from build123d import *

# Parameters (mm, degrees)
ESBO_O1_W             = 42
ESBO_O1_H             = 42
FLANGE_BASE1_DEPTH    = 9.55
CORTE_EXTRUS_O2_DEPTH = 32.196193678
ESBO_O4_R             = 4.8
CORTE_EXTRUS_O4_DEPTH = 32.196193678
ESBO_O16_R            = 2
CORTE_EXTRUS_O6_DEPTH = 3
ESBO_O19_R            = 1.6
CORTE_EXTRUS_O7_DEPTH = 31.412209719


# Sheet-metal steps are written as plain solids
with BuildPart() as part:
    # Esboço1 → Flange-base1 (new body)
    with BuildSketch(Plane(origin=(0, 0, 0), x_dir=(1, 0, 0), z_dir=(0, 1, 0))):
        Rectangle(ESBO_O1_W, ESBO_O1_H)
    extrude(amount=-FLANGE_BASE1_DEPTH)

    # Esboço3 → Corte-extrusão2 (cut, through all)
    with BuildSketch(Plane.XZ.offset(9.55)):
        Polygon((-21, 16.757359313), (-16.757359313, 21), (-21, 21), align=None)
        Polygon((-21, -21), (-21, -16.757359313), (-16.757359313, -21), align=None)
        Polygon((21, -21), (21, -16.757359313), (16.757359313, -21), align=None)
        Polygon((21, 16.757359313), (21, 21), (16.757359313, 21), align=None)
    extrude(amount=-CORTE_EXTRUS_O2_DEPTH, mode=Mode.SUBTRACT)

    # Esboço4 → Corte-extrusão4 (cut, through all)
    with BuildSketch(Plane.XZ.offset(9.55)):
        with Locations(Location((0, 0, 0), (0, 0, 270))):
            Circle(ESBO_O4_R)
    extrude(amount=-CORTE_EXTRUS_O4_DEPTH, mode=Mode.SUBTRACT)

    # Esboço16 → Corte-extrusão6 (cut)
    with BuildSketch(Plane.XZ.offset(9.55)):
        with Locations(Location((-15.5, -15.5, 0), (0, 0, 270))):
            Circle(ESBO_O16_R)
        with Locations(Location((-15.5, 15.5, 0), (0, 0, 270))):
            Circle(ESBO_O16_R)
        with Locations(Location((15.5, 15.5, 0), (0, 0, 270))):
            Circle(ESBO_O16_R)
        with Locations(Location((15.5, -15.5, 0), (0, 0, 270))):
            Circle(ESBO_O16_R)
    extrude(amount=-CORTE_EXTRUS_O6_DEPTH, mode=Mode.SUBTRACT)

    # Esboço19 → Corte-extrusão7 (cut, through all)
    with BuildSketch(Plane.XZ.offset(6.55)):
        with Locations(Location((15.5, -15.5, 0), (0, 0, 270))):
            Circle(ESBO_O19_R)
        with Locations(Location((-15.5, -15.5, 0), (0, 0, 270))):
            Circle(ESBO_O19_R)
        with Locations(Location((15.5, 15.5, 0), (0, 0, 270))):
            Circle(ESBO_O19_R)
        with Locations(Location((-15.5, 15.5, 0), (0, 0, 270))):
            Circle(ESBO_O19_R)
    extrude(amount=-CORTE_EXTRUS_O7_DEPTH, mode=Mode.SUBTRACT)


solid = part.part
Geometry check sheet. Reference: the model listing, model coordinates, mm. A direction names the side the tool comes from. Round coordinates to 2 decimals unless told otherwise and drop trailing zeros. Write each loop counter-clockwise with the first axis right and the second up, starting at its lowest first coordinate (ties: lowest second). Pieces come first, ordered by that corner, then holes. Notation, with made-up numbers: (6, 34.25) -> (35, 34.25) arc R8 ccw to (35, 42.25) -> close; hole circle Ø8 at (36.25, 83). An arc over 180 degrees is marked (long way). One line per item, written item: value. Start each with the question number.
(1) Go/stop test with flat-tipped pins: pin 1 Ø11 at (x, z) = (0, 0) entering from -Y; pin 2 Ø3.5 at (x, z) = (15.5, 15.5) entering from -Y; pin 3 Ø1.2 at (x, z) = (16, 16) entering from -Y (3 decimals); pin 4 Ø1.2 at (x, z) = (-15, 16.5) entering from -Y. Record where each tip stops, or that it passes through.
(2) Access from +Z, -Z, +X, -X, +Y, -Y to the whole of each face (thin tool, end or side, straight path). Record for faces 1 (the cylindrical face through (-13.517, -8.071, -15.24)), 2 (the flat face through (-21, -5, 0)).
(3) Scan lines: line 1 (X direction, y = -3, z = -15.5); line 2 (X direction, y = -8.9, z = 15.5); line 3 (Z direction, x = -14.5, y = -7.75). Record each from-to range of solid material in increasing order. Write a range as [from, to].
(4) Cross-section at B-B, the plane z = -15.5. Record the cut outline in (x, y), and give its area (3 significant figures).
(5) Cross-section at C-C, the plane y = -3.75. Record the cut outline in (x, z).
(6) Cross-section at A-A, the plane x = -15.5. Record the cut outline in (y, z), and give its area (3 significant figures).
(7) Cross-section at D-D, the plane x = -2.5. Record the cut outline in (y, z).
(8) Draft check along X on faces 3 (the cylindrical face through (16.58, -3.32, 16.68)), 4 (the flat face through (18.91, -4.84, -18.85)), 5 (the flat face through (-18.91, -4.84, 18.85)). Enter one of: +X half, -X half, draft (parallel to the pull), parting line (faces both ways), or undercut.
Answer:
1. pin 1: y = -9.55
1. pin 2: y = -6.55
1. pin 3: through
1. pin 4: y = -6.55
2. face 1: -Y
2. face 2: +Z, -Z, -X, +Y, -Y
3. line 1: [-21, -17.1], [-13.9, 13.9], [17.1, 21]
3. line 2: [-21, -17.5], [-13.5, 13.5], [17.5, 21]
3. line 3: [-21, -17.23], [-13.77, 13.77], [17.23, 21]
4. outline: (-21, -9.55) -> (-17.5, -9.55) -> (-17.5, -6.55) -> (-17.1, -6.55) -> (-17.1, 0) -> (-21, 0) -> close; (-13.9, -6.55) -> (-13.5, -6.55) -> (-13.5, -9.55) -> (13.5, -9.55) -> (13.5, -6.55) -> (13.9, -6.55) -> (13.9, 0) -> (-13.9, 0) -> close; (17.1, -6.55) -> (17.5, -6.55) -> (17.5, -9.55) -> (21, -9.55) -> (21, 0) -> (17.1, 0) -> close
4. area: 335 mm²
5. outline: (-21, -16.76) -> (-16.76, -21) -> (16.76, -21) -> (21, -16.76) -> (21, 16.76) -> (16.76, 21) -> (-16.76, 21) -> (-21, 16.76) -> close; hole circle Ø3.2 at (-15.5, -15.5); hole circle Ø3.2 at (-15.5, 15.5); hole circle Ø9.6 at (0, 0); hole circle Ø3.2 at (15.5, -15.5); hole circle Ø3.2 at (15.5, 15.5)
6. outline: (-9.55, -21) -> (0, -21) -> (0, -17.1) -> (-6.55, -17.1) -> (-6.55, -17.5) -> (-9.55, -17.5) -> close; (-9.55, -13.5) -> (-6.55, -13.5) -> (-6.55, -13.9) -> (0, -13.9) -> (0, 13.9) -> (-6.55, 13.9) -> (-6.55, 13.5) -> (-9.55, 13.5) -> close; (-9.55, 17.5) -> (-6.55, 17.5) -> (-6.55, 17.1) -> (0, 17.1) -> (0, 21) -> (-9.55, 21) -> close
6. area: 335 mm²
7. outline: (-9.55, -21) -> (0, -21) -> (0, -4.1) -> (-9.55, -4.1) -> close; (-9.55, 4.1) -> (0, 4.1) -> (0, 21) -> (-9.55, 21) -> close
8. face 3: undercut
8. face 4: +X half
8. face 5: -X half
